Could you check a few things on this model? Use its own coordinates, in mm. Give positions to 0.01 mm unless a question says otherwise; leave off trailing zeros. Loops run counter-clockwise (first coordinate to the right, second up) from the corner with the lowest first, then second, coordinate; pieces in that order, holes last. Notation, with made-up numbers: (87, -2) -> (132, -2) arc R11 ccw to (132, 18) -> close; hole circle Ø2 at (28, 72.25). An arc over 180 degrees is marked (long way). Put each result on its own line as item: value.
```python
from build123d import *

# Parameters (mm, degrees)
BOSS_EXTRUDE1_DEPTH     = 250
CUT_EXTRUDE6_DEPTH      = 242
CUT_EXTRUDE6_DEPTH_BACK = 242
SKETCH9_W               = 0.558111167
SKETCH9_H               = 1.818787441
CUT_EXTRUDE7_START      = -8
SKETCH11_R              = 0.139327756
SKETCH11_R_2            = 0.125822814
CUT_EXTRUDE7_DEPTH      = 8
SKETCH13_R              = 0.125822814
CUT_EXTRUDE12_DEPTH     = 1
FILLET3_R               = 0.5


with BuildPart() as part:
    # Sketch1 → Boss-Extrude1 (new, symmetric)
    with BuildSketch(Plane.XY):
        with BuildLine():
            Line((2.869208069, 3.068545431), (-3.706559837, 3.068545431))
            Line((-3.706559837, 3.068545431), (-3.706559837, 2.312213583))
            ThreePointArc((-3.706559837, 2.312213583), (-1.749706829, 0.836593392), (-0.796044874, -1.421117289))
            ThreePointArc((-0.796044874, -1.421117289), (-0.61902671, -1.745895622), (-0.271314784, -1.872041617))
            ThreePointArc((-0.271314784, -1.872041617), (0, -1.870162722), (0.271314784, -1.872041617))
            ThreePointArc((0.271314784, -1.872041617), (0.61902671, -1.745895622), (0.796044874, -1.421117289))
            ThreePointArc((0.796044874, -1.421117289), (1.477625841, 0.448969612), (2.869208069, 1.872091721))
            Line((2.869208069, 1.872091721), (2.869208069, 3.068545431))
        make_face()
    extrude(amount=BOSS_EXTRUDE1_DEPTH, both=True)

    # Sketch9 → Cut-Extrude6 (cut, two sides: drawn at the far end of the back side and taken through both)
    with BuildSketch(Plane.XY.offset(-CUT_EXTRUDE6_DEPTH_BACK)):
        with Locations((2.590152485, 2.15915171)):
            Rectangle(SKETCH9_W, SKETCH9_H)
    extrude(amount=CUT_EXTRUDE6_DEPTH + CUT_EXTRUDE6_DEPTH_BACK, mode=Mode.SUBTRACT)

    # Sketch11 → Cut-Extrude7 (cut)
    # profile 1 of 2: a face of its own
    with BuildSketch(Plane(origin=(0, 0, 242), x_dir=(-1, 0, 0), z_dir=(0, 0, -1)).offset(CUT_EXTRUDE7_START)):
        with Locations((-2.619208069, 2.568545431)):
            Circle(SKETCH11_R)
    # profile 2 of 2: a face of its own
    with BuildSketch(Plane(origin=(0, 0, 242), x_dir=(-1, 0, 0), z_dir=(0, 0, -1)).offset(CUT_EXTRUDE7_START)):
        with BuildLine():
            Line((3.706559837, 3.068545431), (3.706559837, 2.312213583))
            ThreePointArc((3.706559837, 2.312213583), (3.423086279, 2.186837068), (3.14844867, 2.043133511))
            Line((3.14844867, 2.043133511), (3.14844867, 3.068545431))
            Line((3.14844867, 3.068545431), (3.706559837, 3.068545431))
        make_face()
        with Locations((3.438785788, 2.465008687)):
            Circle(SKETCH11_R_2, mode=Mode.SUBTRACT)
    cut_extrude7 = extrude(amount=CUT_EXTRUDE7_DEPTH, mode=Mode.SUBTRACT)

    # Sketch13 → Cut-Extrude12 (cut)
    with BuildSketch(Plane.XY.offset(250)):
        with Locations(Location((-3.438785788, 2.465008687, 0), (0, 0, 180))):
            Circle(SKETCH13_R)
    cut_extrude12 = extrude(amount=-CUT_EXTRUDE12_DEPTH, mode=Mode.SUBTRACT)

    # Mirror1: Cut-Extrude7, Cut-Extrude12 across plane
    add(cut_extrude7.mirror(Plane.XY), mode=Mode.SUBTRACT)
    add(cut_extrude12.mirror(Plane.XY), mode=Mode.SUBTRACT)

    # Fillet3
    fillet3_edges = [part.edges().sort_by_distance(p)[0] for p in [
        (-3.14844867, 2.043133511, -246),
        (2.869208069, 1.872091721, 246),
        (2.869208069, 1.872091721, -246),
        (2.311096902, 1.439762425, 0),
        (-3.706559837, 2.312213583, 0),
        (-3.14844867, 2.043133511, 246),
    ]]
    fillet(fillet3_edges, radius=FILLET3_R)


solid = part.part
```
1. If we section it at A-A (z = 50.5): List the corners of the cut face in (x, y) for me.
Recorded:
outline: (-3.71, 2.64) arc R0.5 ccw to (-3.42, 2.19) arc R4.72 cw to (-0.8, -1.42) arc R0.52 ccw to (-0.27, -1.87) arc R19.59 cw to (0.27, -1.87) arc R0.52 ccw to (0.8, -1.42) arc R4.72 cw to (2.16, 1.3) arc R0.5 ccw to (2.31, 1.66) -> (2.31, 3.07) -> (-3.71, 3.07) -> close
2. If we section it at B-B (y = 0.55): List the corners of the cut face in (x, z) for me, then the cut area to 3 significant figures.
Recorded:
outline: (-1.54, -250) -> (1.54, -250) -> (1.54, 250) -> (-1.54, 250) -> close
area: 1,540 mm^2
3. I need wall thicknesses on line 1 (Y direction, x = -2.25, z = 89.5); line 2 (Y direction, x = -2.75, z = -51.5); line 3 (X direction, y = -1.3, z = -208.5). Which ranges of each line are inside material? Lowest first, please.
Recorded:
line 1: y = 1.38 to 3.07
line 2: y = 1.79 to 3.07
line 3: x = -0.81 to 0.81
4. I'm going to push flat-ended pins straight in: pin 1 (1.6 mm diameter, centred on y = 2.5, z = -14, fed in from +X); pin 2 (2 mm diameter, centred on y = 0, z = -162.5, fed in from +X). Where does each tip first touch, or does it pass through?
Recorded:
pin 1: stops at x = 2.31
pin 2: stops at x = 1.88
